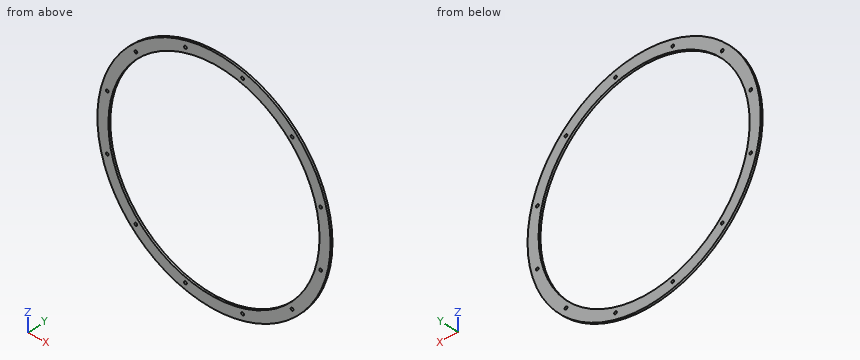
from build123d import *

# Parameters (mm, degrees)
SCHIZZO1_R                   = 258
SCHIZZO1_R_2                 = 3.4
ESTRUSIONE_ESTRUSIONE1_DEPTH = 2.5


with BuildPart() as part:
    # Schizzo1 → Estrusione-Estrusione1 (new, symmetric)
    with BuildSketch(Plane(origin=(0, 0, 0), x_dir=(1, 0, 0), z_dir=(0, 1, 0))):
        with BuildLine():
            ThreePointArc((-285, 0), (0, -285), (285, 0))
            ThreePointArc((285, 0), (0, 285), (-285, 0))
        make_face()
        with Locations(Location((0, 0, 0), (0, 0, 270))):
            Circle(SCHIZZO1_R, mode=Mode.SUBTRACT)
        with Locations(Location((-260.799973098, 69.881142178, 0), (0, 0, 270))):
            Circle(SCHIZZO1_R_2, mode=Mode.SUBTRACT)
        with Locations(Location((-190.91883092, 190.91883092, 0), (0, 0, 270))):
            Circle(SCHIZZO1_R_2, mode=Mode.SUBTRACT)
        with Locations(Location((-69.881142178, 260.799973098, 0), (0, 0, 270))):
            Circle(SCHIZZO1_R_2, mode=Mode.SUBTRACT)
        with Locations(Location((69.881142178, 260.799973098, 0), (0, 0, 270))):
            Circle(SCHIZZO1_R_2, mode=Mode.SUBTRACT)
        with Locations(Location((190.91883092, 190.91883092, 0), (0, 0, 270))):
            Circle(SCHIZZO1_R_2, mode=Mode.SUBTRACT)
        with Locations(Location((260.799973098, 69.881142178, 0), (0, 0, 270))):
            Circle(SCHIZZO1_R_2, mode=Mode.SUBTRACT)
        with Locations(Location((260.799973098, -69.881142178, 0), (0, 0, 270))):
            Circle(SCHIZZO1_R_2, mode=Mode.SUBTRACT)
        with Locations(Location((190.91883092, -190.91883092, 0), (0, 0, 270))):
            Circle(SCHIZZO1_R_2, mode=Mode.SUBTRACT)
        with Locations(Location((69.881142178, -260.799973098, 0), (0, 0, 270))):
            Circle(SCHIZZO1_R_2, mode=Mode.SUBTRACT)
        with Locations(Location((-69.881142178, -260.799973098, 0), (0, 0, 270))):
            Circle(SCHIZZO1_R_2, mode=Mode.SUBTRACT)
        with Locations(Location((-190.91883092, -190.91883092, 0), (0, 0, 270))):
            Circle(SCHIZZO1_R_2, mode=Mode.SUBTRACT)
        with Locations(Location((-260.799973098, -69.881142178, 0), (0, 0, 270))):
            Circle(SCHIZZO1_R_2, mode=Mode.SUBTRACT)
    extrude(amount=ESTRUSIONE_ESTRUSIONE1_DEPTH, both=True)


solid = part.part
CAD build for the part. Positions are in the model's coordinates, mm. Round coordinates to 2 decimals unless told otherwise and drop trailing zeros. Write each loop counter-clockwise with the first axis right and the second up, starting at its lowest first coordinate (ties: lowest second). Pieces come first, ordered by that corner, then holes. Notation, with made-up numbers: M 11,-16 L 45,-16 A23 cw 45,19 Z; hole C 25,42 d9. An arc over 180 degrees is marked long. Put each result on its own line as item: value. Start each with the question number.
1) Saw through at A-A, the plane x = 0. Write the cut outline in (y, z).
2) Saw through at C-C, the plane y = -0.8. Count the separate pieces of the cut face and the enclosed holes in it, and give its area (3 significant figures).
3) Saw through at B-B, the plane z = -22.5. Write the cut outline in (x, y), and give its area (3 significant figures).
4) Pin check, flat tips, straight feed: pin 1 Ø1.5 at (x, y) = (-203.5, 1) entering from +Z; pin 2 Ø6 at (x, z) = (-69.88, 260.8) entering from +Y; pin 3 Ø2 at (y, z) = (1, 76) entering from +X. Stop position of each tip, or through.
5) Drill centre lines: probe 1 along Z at (x, y) = (-229, -0.65); probe 2 along Z at (x, y) = (199.5, 1.8); probe 3 along X at (y, z) = (0.3, -139.5). Where is each one in solid material? Low to high. Write a range as [from, to].
Resolved:
1. outline: M -2.5,-285 L 2.5,-285 L 2.5,-258 L -2.5,-258 Z; M -2.5,258 L 2.5,258 L 2.5,285 L -2.5,285 Z
2. separate pieces: 1
2. enclosed holes: 13
2. area: 45,600 mm²
3. outline: M -284.11,-2.5 L -257.02,-2.5 L -257.02,2.5 L -284.11,2.5 Z; M 257.02,-2.5 L 284.11,-2.5 L 284.11,2.5 L 257.02,2.5 Z
3. area: 271 mm²
4. pin 1: z = 200.29
4. pin 2: through
4. pin 3: x = 274.95
5. probe 1: [-169.66, -118.84], [118.84, 169.66]
5. probe 2: [-203.53, -163.6], [163.6, 203.53]
5. probe 3: [-248.53, -217.03], [217.03, 248.53]
